Part model, mm, in its own coordinate system. A direction names the side the tool comes from. Give positions to 0.01 mm unless a question says otherwise; leave off trailing zeros. Write each loop counter-clockwise with the first axis right and the second up, starting at its lowest first coordinate (ties: lowest second). Pieces come first, ordered by that corner, then holes. Notation, with made-up numbers: (87, 77.25) - (143, 77.25) arc R24 ccw to (143, 88.25) - close; hole circle Ø7 at (-1.5, -24.5). An arc over 180 degrees is marked (long way). Answer as a JSON object with one key per item and string values. Group by question number.
```python
from build123d import *
from OCP.BRepAlgoAPI import BRepAlgoAPI_Cut
from OCP.TopTools import TopTools_ListOfShape

# Parameters (mm, degrees)
CROQUIS1_R              = 1.500000001
SALIENTE_EXTRUIR1_DEPTH = 3
CROQUIS4_W              = 3
CROQUIS4_H              = 71.0001277
SALIENTE_EXTRUIR2_DEPTH = 15
CROQUIS5_R              = 6.5
CROQUIS5_R_2            = 1.5
CROQUIS5_R_3            = 2.5
CROQUIS5_W              = 2.499996062
CROQUIS5_H              = 6.000001641
CORTAR_EXTRUIR1_DEPTH   = 10
CORTAR_EXTRUIR3_START   = -4
CORTAR_EXTRUIR3_DEPTH   = 5
CROQUIS7_W              = 3
CROQUIS7_H              = 65.000131742
CORTAR_EXTRUIR4_DEPTH   = 9


with BuildPart() as part:
    # Croquis1 → Saliente-Extruir1 (new body)
    with BuildSketch(Plane.XY):
        with BuildLine():
            Line((314.494178041, 188.579504075), (317.494178043, 188.579506619))
            Line((317.494178043, 188.579506619), (317.494186524, 178.579506615))
            Line((317.494186524, 178.579506615), (314.494177731, 178.579504071))
            Line((314.494177731, 178.579504071), (314.494186212, 168.579504067))
            Line((314.494186212, 168.579504067), (317.494186214, 168.579506611))
            Line((317.494186214, 168.579506611), (317.494190454, 163.579648323))
            Line((317.494190454, 163.579648323), (314.494168474, 163.579645778))
            Line((314.494168474, 163.579645778), (314.494176956, 153.579645774))
            Line((314.494176956, 153.579645774), (317.494159374, 153.579648318))
            Line((317.494159374, 153.579648318), (317.494167855, 143.579648314))
            Line((317.494167855, 143.579648314), (314.494167854, 143.57964577))
            Line((314.494167854, 143.57964577), (314.494173605, 130.579645765))
            Line((314.494173605, 130.579645765), (327.013519861, 130.579618443))
            Line((327.013519861, 130.579618443), (327.013522591, 133.579618444))
            Line((327.013522591, 133.579618444), (339.532765197, 133.579591123))
            Line((339.532765197, 133.579591123), (339.532765197, 130.57943755))
            Line((339.532765197, 130.57943755), (348.284914925, 130.579428178))
            Line((348.284914925, 130.579428178), (348.284918137, 133.579395242))
            Line((348.284918137, 133.579395242), (357.034918141, 133.579385871))
            Line((357.034918141, 133.579385871), (357.034914928, 130.57938587))
            ThreePointArc((357.034914928, 130.57938587), (361.414562849, 127.449962294), (365.794217472, 130.57937649))
            Line((365.794217472, 130.57937649), (365.794220685, 133.579299126))
            Line((365.794220685, 133.579299126), (374.544220688, 133.579289756))
            Line((374.544220688, 133.579289756), (374.544217476, 130.579290106))
            Line((374.544217476, 130.579290106), (383.294100119, 130.579288157))
            Line((383.294100119, 130.579288157), (383.294100787, 133.579288158))
            Line((383.294100787, 133.579288158), (395.694123645, 133.579285396))
            Line((395.694123645, 133.579285396), (395.694122977, 130.579285394))
            Line((395.694122977, 130.579285394), (414.49422245, 130.579281206))
            Line((414.49422245, 130.579281206), (414.494175849, 201.579408906))
            Line((414.494175849, 201.579408906), (395.654796079, 201.579436111))
            Line((395.654796079, 201.579436111), (395.654796079, 198.559911251))
            Line((395.654796079, 198.559911251), (383.254781657, 198.559889448))
            Line((383.254781657, 198.559889448), (383.254781657, 201.579454018))
            Line((383.254781657, 201.579454018), (374.544176149, 201.579466597))
            Line((374.544176149, 201.579466597), (374.544170874, 198.579568646))
            Line((374.544170874, 198.579568646), (365.794170871, 198.579584031))
            Line((365.794170871, 198.579584031), (365.794176145, 201.579506668))
            ThreePointArc((365.794176145, 201.579506668), (361.414530376, 204.708933254), (357.034873601, 201.579522069))
            Line((357.034873601, 201.579522069), (357.034868326, 198.579522068))
            Line((357.034868326, 198.579522068), (348.284868323, 198.579537453))
            Line((348.284868323, 198.579537453), (348.284873598, 201.579504517))
            Line((348.284873598, 201.579504517), (339.493492813, 201.579517212))
            Line((339.493492813, 201.579517212), (339.493492813, 198.559812504))
            Line((339.493492813, 198.559812504), (327.093469951, 198.559790701))
            Line((327.093469951, 198.559790701), (327.093469951, 201.579535118))
            Line((327.093469951, 201.579535118), (314.494181082, 201.579553313))
            Line((314.494181082, 201.579553313), (314.494178041, 188.579504075))
        make_face()
        with Locations((361.414522236, 200.079542161)):
            Circle(CROQUIS1_R, mode=Mode.SUBTRACT)
        with Locations((361.414567806, 132.079353387)):
            Circle(CROQUIS1_R, mode=Mode.SUBTRACT)
    extrude(amount=SALIENTE_EXTRUIR1_DEPTH)

    # Croquis4 → Saliente-Extruir2 (add)
    with BuildSketch(Plane(origin=(414.494308155, 0.000272052, 0), x_dir=(0, 0, -1), z_dir=(0.9999999999997846, 6.563478556519826e-07, 0))):
        with Locations((-1.5, 166.079073004)):
            Rectangle(CROQUIS4_W, CROQUIS4_H)
    extrude(amount=SALIENTE_EXTRUIR2_DEPTH)

    # Croquis5 → Cortar-Extruir1 (cut)
    with BuildSketch(Plane.XY.offset(3)):
        with Locations((398.294185249, 187.258674364)):
            Circle(CROQUIS5_R)
        with Locations((377.694190992, 178.508660843)):
            Circle(CROQUIS5_R_2)
        with Locations((377.694179506, 196.008660843)):
            Circle(CROQUIS5_R_2)
        with Locations((387.494185249, 187.258667276)):
            Circle(CROQUIS5_R_3)
        with Locations((366.244185249, 187.258653329)):
            Rectangle(CROQUIS5_W, CROQUIS5_H)
    extrude(amount=-CORTAR_EXTRUIR1_DEPTH, mode=Mode.SUBTRACT)

    # Cortar-Extruir3: read off the stored shape, not the designer's step
    # Cortar-Extruir3 outline → Cortar-Extruir3 (cut)
    with BuildSketch(Plane(origin=(0, 0, 0), x_dir=(-1, 0, 0), z_dir=(0, 0, -1)).offset(CORTAR_EXTRUIR3_START)):
        Polygon((-429.494175849, 201.579418751), (-429.494177818, 198.579417138), (-408.794180476, 198.579417138), (-408.794180476, 201.579418751), (-414.494175849, 201.579408906), align=None)
        Polygon((-408.79422983, 133.579285396), (-429.49422245, 133.579285396), (-429.49422245, 130.579291051), (-414.49422245, 130.579281206), (-408.79422983, 130.579282476), align=None)
    extrude(amount=CORTAR_EXTRUIR3_DEPTH, mode=Mode.SUBTRACT)


with BuildPart() as cortar_extruir4_tool:
    # Croquis7 → Cortar-Extruir4 (new body)
    with BuildSketch(Plane(origin=(429.494308155, 0.000281898, 0), x_dir=(0, 0, -1), z_dir=(0.9999999999997846, 6.563478556519826e-07, 0))):
        with Locations((-1.5, 166.079069369)):
            Rectangle(CROQUIS7_W, CROQUIS7_H)
    extrude(amount=-CORTAR_EXTRUIR4_DEPTH)


with BuildPart() as part_1:
    add(part.part)

    # Cortar-Extruir4: cut by cortar_extruir4_tool, with a tolerance
    cortar_extruir4_stock = TopTools_ListOfShape()
    cortar_extruir4_stock.Append(part_1.part.wrapped)
    cortar_extruir4_tools = TopTools_ListOfShape()
    cortar_extruir4_tools.Append(cortar_extruir4_tool.part.wrapped)
    cortar_extruir4_cut = BRepAlgoAPI_Cut()
    cortar_extruir4_cut.SetArguments(cortar_extruir4_stock)
    cortar_extruir4_cut.SetTools(cortar_extruir4_tools)
    cortar_extruir4_cut.SetFuzzyValue(0.00001)
    cortar_extruir4_cut.Build()
    add(Compound.cast(cortar_extruir4_cut.Shape()).solids(), mode=Mode.REPLACE)


solid = part_1.part
```
1) Band-saw the part on A-A (y = 186). List the corners of the cut face in (x, z).
2) Band-saw the part on C-C (y = 149). List the corners of the cut face in (x, z), plus the area to 3 significant figures.
3) Band-saw the part on B-B (x = 381). List the corners of the cut face in (y, z).
4) Drop flat-ended pins along their axis: P1, Ø0.9, axis at x = 315.5, z = 1.5, coming from the +Y side; P2, Ø10, axis at x = 351.5, y = 191, coming from the -Z side; P3, Ø0.9, axis at y = 200, z = 2, coming from the +X side; P4, Ø1.5, axis at x = 344, z = 2, coming from the -Y side. Give the stop position or say it passes through.
5) Which spindle directions (+Z, -Z, +X, -X, +Y, -Y) get a long thin tool onto all of the face, cutting with end or side? Do faces 1 (the flat face through (316, 188.58, 1)), 2 (the flat face through (379, 130.579, 1)), 3 (the flat face through (383.255, 200, 1)), 4 (the flat face through (383.294, 132, 1)), 5 (the flat face through (364.994, 187, 2)). Say none if no direction does.
6) Mould opens along Y. For faces 6 (the flat face through (339.533, 132, 1)), 7 (the flat face through (389, 133.579, 1)), 8 (the flat face through (316, 178.58, 1)) say: pulls with the +Y half, pulls with the -Y half, needs draft (parallel to the pull), parting line crosses it, or undercut.
7) Probe line 1 (Y direction, x = 387.5, z = 2.6); line 2 (Y direction, x = 361, z = 1.25); line 3 (Y direction, x = 341, z = 0.85). List the from-to ranges inside material, lowest first.
8) Band-saw the part on D-D (z = 2.35). State how many separate pieces and enclosed holes the cut face has, plus the area to 3 significant figures.
Verdict:
{
 "1": {"outline": "(317.49, 0) - (364.99, 0) - (364.99, 3) - (317.49, 3) - close; (367.49, 0) - (385.33, 0) - (385.33, 3) - (367.49, 3) - close; (389.65, 0) - (391.92, 0) - (391.92, 3) - (389.65, 3) - close; (404.67, 0) - (420.49, 0) - (420.49, 3) - (404.67, 3) - close"},
 "2": {"outline": "(317.49, 0) - (420.49, 0) - (420.49, 3) - (317.49, 3) - close", "area": "309 mm2"},
 "3": {"outline": "(130.58, 0) - (201.58, 0) - (201.58, 3) - (130.58, 3) - close"},
 "4": {"P1": "y = 201.58", "P2": "z = 0", "P3": "x = 408.79", "P4": "y = 130.58"},
 "5": {"face 1": "+Z, -Z, -X", "face 2": "+Z, -Z, +X, -Y", "face 3": "+Z, -Z, +Y", "face 4": "+Z, -Z, -Y", "face 5": "+Z, -Z"},
 "6": {"face 6": "needs draft", "face 7": "pulls with the -Y half", "face 8": "undercut"},
 "7": {"line 1": "133.58 to 184.76, 189.76 to 198.56", "line 2": "127.47 to 130.64, 133.52 to 198.64, 201.52 to 204.69", "line 3": "130.58 to 201.58"},
 "8": {"separate pieces": "1", "enclosed holes": "7", "area": "6,970 mm2"}
}
